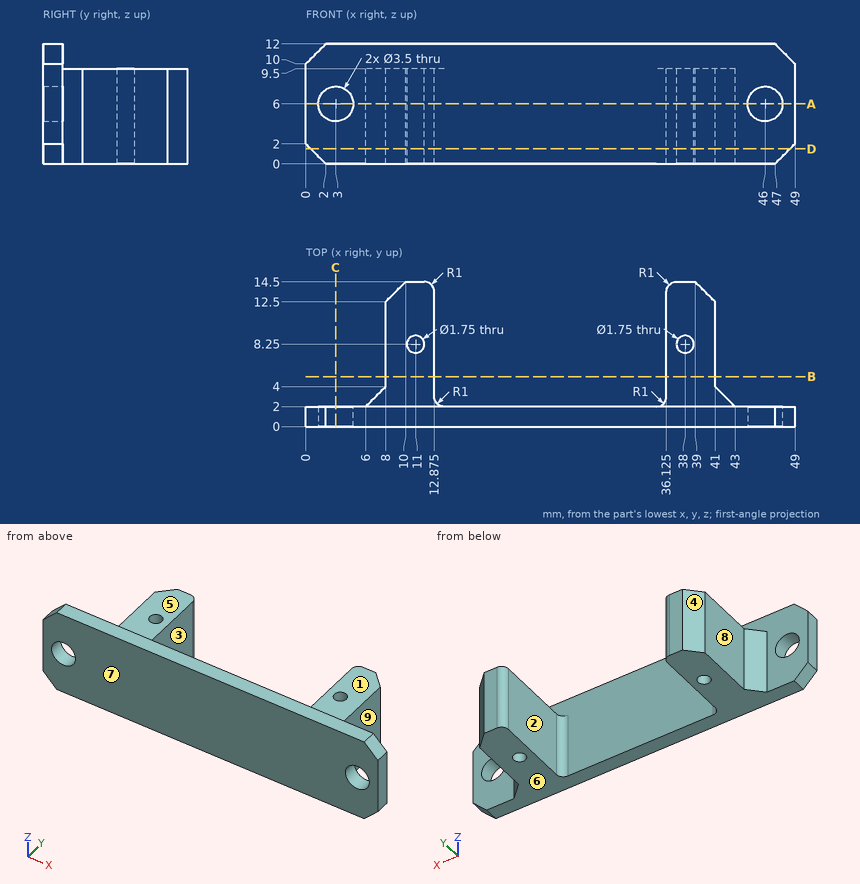
Geometry check sheet. Reference: drawing and pictorial views, mm from the part's lowest x, y, z. A direction names the side the tool comes from. Round coordinates to 2 decimals unless told otherwise and drop trailing zeros. Loops run counter-clockwise (first coordinate to the right, second up) from the corner with the lowest first, then second, coordinate; pieces in that order, holes last. Notation, with made-up numbers: (45, 31.5) -> (63, 31.5) arc R11 cw to (63, 46.5) -> close; hole circle Ø8 at (8, 63.5). An arc over 180 degrees is marked (long way). Answer as a JSON object with one key per item and string values. Group by question number.
Item 1: Cross-section at A-A, the plane z = 6. Count the separate pieces of the cut face and the enclosed holes in it, plus the area to 3 significant figures.
Item 2: Cross-section at D-D, the plane z = 1.5. Record the cut outline in (x, y) (3 decimals), plus the area to 3 significant figures.
Item 3: Release check for a two-part mould opening along X. For the marked faces 1, 2, 3 and 4 record: pulls with the +X half, pulls with the -X half, needs draft (parallel to the pull), parting line crosses it, or undercut.
Item 4: Set-up check for the marked faces 5, 6, 7, 8 and 9: record each of +Z, -Z, +X, -X, +Y, -Y from which the full face is reachable in a straight line by a thin tool's end or side.
Item 5: Thickness scan on line 1 along Z through (x, y) = (3, 0.75); line 2 along X through (y, z) = (10.5, 3) (3 decimals); line 3 along Y through (x, z) = (38, 3) (3 decimals). Record the ranges inside material, lowest first.
Item 6: Depth check by flat-ended pin: pin 1 Ø5.5 at (x, z) = (3, 6) entering from +Y; pin 2 Ø2 at (y, z) = (3.5, 7.5) entering from +X; pin 3 Ø1.4 at (x, y) = (38, 8.25) entering from -Z; pin 4 Ø5 at (y, z) = (7, 4) entering from +X. Enter the tip coordinate at first touch or a pass-through.
Item 7: Cross-section at B-B, the plane y = 5. Record the cut outline in (x, z) (3 decimals).
Item 8: Cross-section at C-C, the plane x = 3. Record the cut outline in (y, z), plus the area to 3 significant figures.
Determined:
{
 "1": {"separate pieces": "3", "enclosed holes": "2", "area": "201 mm²"},
 "2": {"outline": "(0.5, 0) -> (48.5, 0) -> (48.5, 2) -> (43, 2) -> (41, 4) -> (41, 12.5) -> (39, 14.5) -> (37.125, 14.5) arc R1 ccw to (36.125, 13.5) -> (36.125, 3) arc R1 cw to (35.125, 2) -> (13.875, 2) arc R1 cw to (12.875, 3) -> (12.875, 13.5) arc R1 ccw to (11.875, 14.5) -> (10, 14.5) -> (8, 12.5) -> (8, 4) -> (6, 2) -> (0.5, 2) -> close; hole circle Ø1.75 at (11, 8.25); hole circle Ø1.75 at (38, 8.25)", "area": "213 mm²"},
 "3": {"face 1": "needs draft", "face 2": "undercut", "face 3": "undercut", "face 4": "pulls with the -X half"},
 "4": {"face 5": "+Z, +X, -X, +Y", "face 6": "-Z, +X, -X, +Y, -Y", "face 7": "+Z, -Z, +X, -X, -Y", "face 8": "+Z, -Z, -X, +Y", "face 9": "+Z, -Z, +X, +Y"},
 "5": {"line 1": "z = 0 to 4.25, 7.75 to 12", "line 2": "x = 8 to 12.875, 36.125 to 41", "line 3": "y = 0 to 7.375, 9.125 to 14.5"},
 "6": {"pin 1": "stops at y = 2", "pin 2": "stops at x = 42.5", "pin 3": "passes through", "pin 4": "stops at x = 41"},
 "7": {"outline": "(8, 0) -> (12.875, 0) -> (12.875, 9.5) -> (8, 9.5) -> close; (36.125, 0) -> (41, 0) -> (41, 9.5) -> (36.125, 9.5) -> close"},
 "8": {"outline": "(0, 0) -> (2, 0) -> (2, 4.25) -> (0, 4.25) -> close; (0, 7.75) -> (2, 7.75) -> (2, 12) -> (0, 12) -> close", "area": "17.0 mm²"}
}
